For this review, use the dimensioned drawing (mm, ordinates from the lowest corner) and the shaded views. A direction names the side the tool comes from. Give positions to 0.01 mm unless a question says otherwise; leave off trailing zeros. Write each loop counter-clockwise with the first axis right and the second up, starting at its lowest first coordinate (ties: lowest second). Pieces come first, ordered by that corner, then holes. Notation, with made-up numbers: M 32.5,-35.5 L 58.5,-35.5 A26 cw 58.5,-1.5 Z; hole C 64.5,87 d10. An arc over 180 degrees is marked long. Use a Markdown table: item, result. Add a question column.
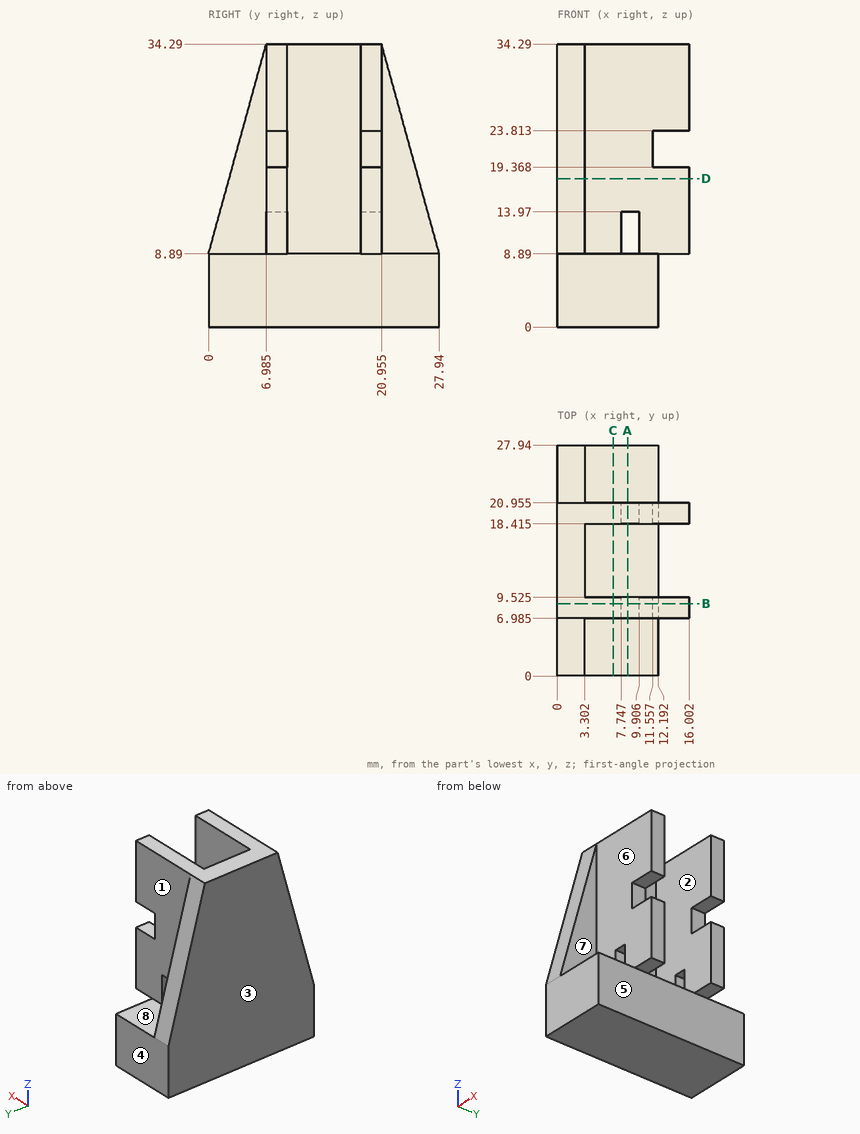
(1) Add section C-C on x = 6.75. Give the boundary of the cut face in (y, z) (1 decimal).
(2) Add section A-A on x = 8.5. Give the boundary of the cut face in (y, z) (1 decimal).
(3) Machinability: for the marked faces 1, 2, 3, 4 and 5, which of the approach directions +Z, -Z, +X, -X, +Y, -Y give a long, thin tool a straight path to every point of the face, cutting with its end or side? Answer none if there is none.
(4) Add section D-D on z = 18. Give the boundary of the cut face in (x, y) (1 decimal), then the cut area to 3 significant figures.
(5) For pin 1 (1 mm diameter, centred on y = 5.5, z = 6.5, fed in from +X); pin 2 (0.8 mm diameter, centred on y = 8, z = 21, fed in from +X); pin 3 (3 mm diameter, centred on x = 13.5, y = 20.5, fed in from -Z); pin 4 (2 mm diameter, centred on x = 14.5, y = 7.5, fed in from -Z), all flat-tipped, find the tip position at first contact; note any pin that passes through.
(6) Wall thickness on L1, parallel to Y at x = 15, z = 19 (1 decimal); L2, parallel to X at y = 8.25, z = 12 (1 decimal); L3, parallel to X at y = 4, z = 11.5: over which ranges is each line inside the solid? List them lowest first.
(7) Add section B-B on y = 8.75. Give the boundary of the cut face in (x, z) (1 decimal), then the cut area to 3 significant figures.
(8) The part is to be moulded in two halves that separate along Y. For the marked faces 6, 7 and 8, say which applies: released by +Y, released by -Y, zero draft, split by the parting line, or undercut.
From the geometry:
| question | item | result |
|---|---|---|
| 1 | outline | M 0,0 L 27.9,0 L 27.9,8.9 L 21,8.9 L 21,34.3 L 18.4,34.3 L 18.4,8.9 L 9.5,8.9 L 9.5,34.3 L 7,34.3 L 7,8.9 L 0,8.9 Z |
| 2 | outline | M 0,0 L 27.9,0 L 27.9,8.9 L 0,8.9 Z; M 7,14 L 9.5,14 L 9.5,34.3 L 7,34.3 Z; M 18.4,14 L 21,14 L 21,34.3 L 18.4,34.3 Z |
| 3 | face 1 | +Z, +X, +Y |
| 3 | face 2 | +Z, +X |
| 3 | face 3 | +Z, -Z, -X, +Y, -Y |
| 3 | face 4 | +Z, -Z, +X, -X, +Y |
| 3 | face 5 | -Z, +X, +Y, -Y |
| 4 | outline | M 0,2.5 L 3.3,2.5 L 3.3,7 L 16,7 L 16,9.5 L 3.3,9.5 L 3.3,18.4 L 16,18.4 L 16,21 L 3.3,21 L 3.3,25.4 L 0,25.4 Z |
| 4 | area | 140 mm^2 |
| 5 | pin 1 | stops at x = 12.19 |
| 5 | pin 2 | stops at x = 11.56 |
| 5 | pin 3 | stops at z = 0 |
| 5 | pin 4 | stops at z = 8.89 |
| 6 | L1 | y = 7 to 9.5, 18.4 to 21 |
| 6 | L2 | x = 0 to 7.7, 9.9 to 16 |
| 6 | L3 | x = 0 to 3.3 |
| 7 | outline | M 0,0 L 12.2,0 L 12.2,8.9 L 16,8.9 L 16,19.4 L 11.6,19.4 L 11.6,23.8 L 16,23.8 L 16,34.3 L 0,34.3 Z; hole M 7.7,8.9 L 9.9,8.9 L 9.9,14 L 7.7,14 Z |
| 7 | area | 484 mm^2 |
| 8 | face 6 | released by -Y |
| 8 | face 7 | zero draft |
| 8 | face 8 | undercut |
